Read the model definition and answer for the solid it produces. Units are mm, in the model's axes. A direction names the side the tool comes from. Give positions to 0.01 mm unless a question says otherwise; leave off trailing zeros. Order: outer loops, then holes, each group sorted by start corner. A loop starts at its lowest first (then second) coordinate and runs counter-clockwise, first axis right, second up. Notation, with made-up numbers: (53, -4) - (57, -4) arc R9 cw to (57, 2) - close; hole circle Ø1 at (64, 75.25). An arc over 180 degrees is marked (long way). One line per item, written item: value. Start each with the question number.
```python
from build123d import *

# Parameters (mm, degrees)
SKETCH1_R           = 1.6
BOSS_EXTRUDE1_DEPTH = 8
CHAMFER1_SIZE       = 1
SKETCH2_R           = 1.6
BOSS_EXTRUDE3_DEPTH = 8
FILLET1_R           = 10
CHAMFER2_SIZE       = 1
CHAMFER3_SIZE       = 1
SKETCH3_R           = 1.6
BOSS_EXTRUDE4_DEPTH = 8
CHAMFER5_SIZE       = 1
FILLET2_R           = 10


with BuildPart() as part:
    # Sketch1 → Boss-Extrude1 (new body)
    with BuildSketch(Plane.XY):
        with BuildLine():
            Line((-0.5, 3), (45.5, 3))
            ThreePointArc((45.5, 3), (47.267766953, 2.267766953), (48, 0.5))
            Line((48, 0.5), (48, -0.5))
            ThreePointArc((48, -0.5), (47.267766953, -2.267766953), (45.5, -3))
            Line((45.5, -3), (-0.5, -3))
            ThreePointArc((-0.5, -3), (-2.267766953, -2.267766953), (-3, -0.5))
            Line((-3, -0.5), (-3, 0.5))
            ThreePointArc((-3, 0.5), (-2.267766953, 2.267766953), (-0.5, 3))
        make_face()
        Circle(SKETCH1_R, mode=Mode.SUBTRACT)
        with Locations((7.5, 0)):
            Circle(SKETCH1_R, mode=Mode.SUBTRACT)
        with Locations((15, 0)):
            Circle(SKETCH1_R, mode=Mode.SUBTRACT)
        with Locations((22.5, 0)):
            Circle(SKETCH1_R, mode=Mode.SUBTRACT)
        with Locations((30, 0)):
            Circle(SKETCH1_R, mode=Mode.SUBTRACT)
        with Locations((37.5, 0)):
            Circle(SKETCH1_R, mode=Mode.SUBTRACT)
        with Locations((45, 0)):
            Circle(SKETCH1_R, mode=Mode.SUBTRACT)
    extrude(amount=BOSS_EXTRUDE1_DEPTH)

    # Chamfer1
    chamfer1_edges = [part.edges().sort_by_distance(p)[0] for p in [
        (-1.6, 0, 0),
        (-1.6, 0, 8),
        (5.9, 0, 0),
        (5.9, 0, 8),
        (13.4, 0, 0),
        (13.4, 0, 8),
        (20.9, 0, 0),
        (20.9, 0, 8),
        (28.4, 0, 0),
        (28.4, 0, 8),
    ]]
    chamfer(chamfer1_edges, length=CHAMFER1_SIZE)

    # Sketch2 → Boss-Extrude3 (add)
    with BuildSketch(Plane.XY.offset(8)):
        with BuildLine():
            ThreePointArc((-3, 0.5), (-2.809698831, 1.456708581), (-2.267766953, 2.267766953))
            Line((-2.267766953, 2.267766953), (-18.529200529, -13.993666623))
            ThreePointArc((-18.529200529, -13.993666623), (-19.261433576, -15.761433576), (-18.529200529, -17.529200529))
            Line((-18.529200529, -17.529200529), (-17.822093748, -18.23630731))
            ThreePointArc((-17.822093748, -18.23630731), (-16.054326795, -18.968540357), (-14.286559842, -18.23630731))
            Line((-14.286559842, -18.23630731), (0.949747468, -3))
            Line((0.949747468, -3), (-0.5, -3))
            ThreePointArc((-0.5, -3), (-2.267766953, -2.267766953), (-3, -0.5))
            Line((-3, -0.5), (-3, 0.5))
        make_face()
        with Locations((-16.054326795, -15.761433576)):
            Circle(SKETCH2_R, mode=Mode.SUBTRACT)
        with Locations((-10.751025936, -10.458132717)):
            Circle(SKETCH2_R, mode=Mode.SUBTRACT)
        with Locations((-5.447725077, -5.154831858)):
            Circle(SKETCH2_R, mode=Mode.SUBTRACT)
    extrude(amount=-BOSS_EXTRUDE3_DEPTH)

    # Fillet1
    fillet1_edges = [part.edges().sort_by_distance(p)[0] for p in [
        (0.949747468, -3, 4),
    ]]
    fillet(fillet1_edges, radius=FILLET1_R)

    # Chamfer2
    chamfer2_edges = [part.edges().sort_by_distance(p)[0] for p in [
        (-17.654326795, -15.761433576, 8),
        (-12.351025936, -10.458132717, 8),
        (-7.047725077, -5.154831858, 8),
        (-7.047725077, -5.154831858, 0),
        (-12.351025936, -10.458132717, 0),
        (-17.654326795, -15.761433576, 0),
    ]]
    chamfer(chamfer2_edges, length=CHAMFER2_SIZE)

    # Chamfer3
    chamfer3_edges = [part.edges().sort_by_distance(p)[0] for p in [
        (35.9, 0, 0),
        (35.9, 0, 8),
        (43.4, 0, 0),
        (43.4, 0, 8),
    ]]
    chamfer(chamfer3_edges, length=CHAMFER3_SIZE)

    # Sketch3 → Boss-Extrude4 (add)
    with BuildSketch(Plane.XY.offset(8)):
        with BuildLine():
            ThreePointArc((-18.529200529, -17.529200529), (-19.071132407, -16.718142157), (-19.261433576, -15.761433576))
            Line((-19.261433576, -15.761433576), (-19.261433576, -37.761433576))
            ThreePointArc((-19.261433576, -37.761433576), (-18.529200529, -39.529200529), (-16.761433576, -40.261433576))
            Line((-16.761433576, -40.261433576), (-15.761433576, -40.261433576))
            ThreePointArc((-15.761433576, -40.261433576), (-13.993666623, -39.529200529), (-13.261433576, -37.761433576))
            Line((-13.261433576, -37.761433576), (-13.261433576, -17.211181044))
            Line((-13.261433576, -17.211181044), (-14.286559842, -18.23630731))
            ThreePointArc((-14.286559842, -18.23630731), (-16.054326795, -18.968540357), (-17.822093748, -18.23630731))
            Line((-17.822093748, -18.23630731), (-18.529200529, -17.529200529))
        make_face()
        with Locations((-16.261433576, -30.261433576)):
            Circle(SKETCH3_R, mode=Mode.SUBTRACT)
        with Locations((-16.261433576, -37.261433576)):
            Circle(SKETCH3_R, mode=Mode.SUBTRACT)
        with Locations((-16.261433576, -23.261433576)):
            Circle(SKETCH3_R, mode=Mode.SUBTRACT)
    extrude(amount=-BOSS_EXTRUDE4_DEPTH)

    # Chamfer5
    chamfer5_edges = [part.edges().sort_by_distance(p)[0] for p in [
        (-17.861433576, -37.261433576, 8),
        (-17.861433576, -30.261433576, 8),
        (-17.861433576, -23.261433576, 8),
        (-17.861433576, -23.261433576, 0),
        (-17.861433576, -30.261433576, 0),
        (-17.861433576, -37.261433576, 0),
    ]]
    chamfer(chamfer5_edges, length=CHAMFER5_SIZE)

    # Fillet2
    fillet2_edges = [part.edges().sort_by_distance(p)[0] for p in [
        (-13.261433576, -17.211181044, 4),
    ]]
    fillet(fillet2_edges, radius=FILLET2_R)


solid = part.part
```
1) Each of these flat-tipped pins is pushed along its axis until it touches: pin 1 (1.9 mm diameter, centred on x = -10.75, y = -10.46, fed in from -Z); pin 2 (3 mm diameter, centred on y = -29.5, z = 2.5, fed in from +X); pin 3 (4 mm diameter, centred on x = -16.26, y = -37.26, fed in from -Z); pin 4 (5 mm diameter, centred on x = 37.5, y = 0, fed in from +Z). Where does it stop, or does it pass through?
2) Find the intervals of material crossed by probe 1 along Y at (x, z) = (22.5, 3.3); probe 2 along X at (y, z) = (-28, 5.5); probe 3 along Y at (x, z) = (12, 7), in increasing order. Write a range as from..to.
3) Section B-B on z = 5.75 is taken. Give the number of separate pieces and of enclosed holes in the cut face, plus the area to 3 significant figures.
4) For faces 1 (the cylindrical face through (28.4, 0.07, 3.96)), 2 (the flat face through (26, -3, 4)), determine the directions among +Z, -Z, +X, -X, +Y, -Y from which every point of the face is accessible in a straight line to the end or side of a thin tool.
5) The mould has two halves that part along X. Classify faces 3 (the flat face through (-13.261, -30, 4)), 4 (the cylindrical face through (-1.469, 2.804, 3.944)), 5 (the cylindrical face through (-10.013, -11.878, 4.042)): +X half, -X half, draft (parallel to the pull), parting line (faces both ways), or undercut.
6) Section A-A on x = 30 is taken. Write down the section's boundary in (y, z).
Solved:
1. pin 1: passes through
1. pin 2: stops at x = -13.26
1. pin 3: stops at z = 0.6
1. pin 4: stops at z = 7.9
2. probe 1: y = -3..-1.6, 1.6..3
2. probe 2: x = -19.26..-13.26
2. probe 3: y = -3..3
3. separate pieces: 1
3. enclosed holes: 13
3. area: 465 mm2
4. face 1: +Z, -Z
4. face 2: +Z, -Z, +X, -Y
5. face 3: +X half
5. face 4: -X half
5. face 5: undercut
6. outline: (-3, 0) - (-2.6, 0) - (-1.6, 1) - (-1.6, 7) - (-2.6, 8) - (-3, 8) - close; (1.6, 1) - (2.6, 0) - (3, 0) - (3, 8) - (2.6, 8) - (1.6, 7) - close
